from build123d import *

# Parameters (mm, degrees)
SKETCH1_W           = 44
SKETCH1_H           = 16
BOSS_EXTRUDE1_DEPTH = 10
SKETCH2_R           = 1.7
CUT_EXTRUDE1_DEPTH  = 25
SKETCH3_R           = 1.75
CUT_EXTRUDE2_DEPTH  = 25
CHAMFER1_SIZE       = 5
FILLET1_R           = 2
SKETCH4_R           = 3.5
CUT_EXTRUDE3_DEPTH  = 4


with BuildPart() as part:
    # Sketch1 → Boss-Extrude1 (new body)
    with BuildSketch(Plane.XY):
        Rectangle(SKETCH1_W, SKETCH1_H)
    extrude(amount=BOSS_EXTRUDE1_DEPTH)

    # Sketch2 → Cut-Extrude1 (cut)
    with BuildSketch(Plane.XZ.offset(8)):
        with Locations(Location((-10, 5, 0), (0, 0, 270))):
            Circle(SKETCH2_R)
        with Locations(Location((10, 5, 0), (0, 0, 270))):
            Circle(SKETCH2_R)
    extrude(amount=-CUT_EXTRUDE1_DEPTH, mode=Mode.SUBTRACT)

    # Sketch3 → Cut-Extrude2 (cut)
    with BuildSketch(Plane.XY.offset(10)):
        with Locations((-16, 0)):
            Circle(SKETCH3_R)
        with Locations(Location((16, 0, 0), (0, 0, 180))):
            Circle(SKETCH3_R)
    extrude(amount=-CUT_EXTRUDE2_DEPTH, mode=Mode.SUBTRACT)

    # Chamfer1
    chamfer1_edges = [part.edges().sort_by_distance(p)[0] for p in [
        (22, -8, 5),
        (-22, -8, 5),
    ]]
    chamfer(chamfer1_edges, length=CHAMFER1_SIZE)

    # Fillet1
    fillet1_edges = [part.edges().sort_by_distance(p)[0] for p in [
        (22, -3, 5),
        (-17, -8, 5),
        (17, -8, 5),
        (-22, -3, 5),
    ]]
    fillet(fillet1_edges, radius=FILLET1_R)

    # Sketch4 → Cut-Extrude3 (cut)
    with BuildSketch(Plane.XZ.offset(8)):
        with Locations(Location((10, 5, 0), (0, 0, 270))):
            Circle(SKETCH4_R)
        with Locations(Location((-10, 5, 0), (0, 0, 270))):
            Circle(SKETCH4_R)
    extrude(amount=-CUT_EXTRUDE3_DEPTH, mode=Mode.SUBTRACT)


solid = part.part
Source: CAD feature listing. Evaluate the final solid. Frame: model axes, mm. A direction names the side the tool comes from. Round coordinates to 2 decimals unless told otherwise and drop trailing zeros. Loops run counter-clockwise (first coordinate to the right, second up) from the corner with the lowest first, then second, coordinate; pieces in that order, holes last. Notation, with made-up numbers: (8.5, 63.5) -> (56.5, 63.5) arc R24 ccw to (56.5, 88.5) -> close; hole circle Ø11 at (58.25, 16.5). An arc over 180 degrees is marked (long way). Answer as a JSON object with one key per item and string values. Group by question number.
Q1. Section query D-D (z = 5.5). Output: boundary loops of the cut face in (x, y), plus the area to 3 significant figures.
Q2. Section query B-B (x = 10). Output: boundary loops of the cut face in (y, z).
Q3. Access query for faces 4 (the flat face through (-22, 3, 5)), 5 (the flat face through (-9, -4, 3)). Directions: +Z, -Z, +X, -X, +Y, -Y. A direction counts if a zero-diameter tool reaches every point of the face in a straight line with its end or side. Return the directions, or none.
Q4. Contact query for flat-ended pins moving along their axis: P1, Ø2, axis at y = -6, z = 8.5, coming from the -X side; P2, Ø4, axis at x = -10, z = 5, coming from the -Y side. Output: stop coordinate, or through.
Q5. Section query C-C (z = 1). Output: boundary loops of the cut face in (x, y).
Q6. Mould query, pull axis X, two halves, no side actions, for faces 1 (the cylindrical face through (-14.331, 0.526, 5.07)), 2 (the flat face through (0, 0, 0)), 3 (the cylindrical face through (16.93, -7.85, 5.07)). Classes: pulls with the +X half, pulls with the -X half, needs draft (parallel to the pull), parting line crosses it, or undercut.
Q7. Section query A-A (y = 0). Output: boundary loops of the cut face in (x, z), plus the area to 3 significant figures.
Q8. Ray query, line 1 (X direction, y = -3.5, z = 5.25); line 2 (X direction, y = -7.5, z = 5); line 3 (X direction, y = 1, z = 6). Return the intervals inside material, ascending. Write a range as from..to.
Completed:
{
 "1": {"outline": "(-22, -2.17) arc R2 ccw to (-21.41, -3.59) -> (-17.59, -7.41) arc R2 ccw to (-16.17, -8) -> (-13.46, -8) -> (-13.46, -4) -> (-11.62, -4) -> (-11.62, 8) -> (-22, 8) -> close; (-8.38, -4) -> (-6.54, -4) -> (-6.54, -8) -> (6.54, -8) -> (6.54, -4) -> (8.38, -4) -> (8.38, 8) -> (-8.38, 8) -> close; (11.62, -4) -> (13.46, -4) -> (13.46, -8) -> (16.17, -8) arc R2 ccw to (17.59, -7.41) -> (21.41, -3.59) arc R2 ccw to (22, -2.17) -> (22, 8) -> (11.62, 8) -> close; hole circle Ø3.5 at (-16, 0); hole circle Ø3.5 at (16, 0)", "area": "526 mm²"},
 "2": {"outline": "(-8, 0) -> (8, 0) -> (8, 3.3) -> (-4, 3.3) -> (-4, 1.5) -> (-8, 1.5) -> close; (-8, 8.5) -> (-4, 8.5) -> (-4, 6.7) -> (8, 6.7) -> (8, 10) -> (-8, 10) -> close"},
 "3": {"face 4": "+Z, -Z, -X, +Y, -Y", "face 5": "-Y"},
 "4": {"P1": "x = -20", "P2": "y = -4"},
 "5": {"outline": "(-22, -2.17) arc R2 ccw to (-21.41, -3.59) -> (-17.59, -7.41) arc R2 ccw to (-16.17, -8) -> (16.17, -8) arc R2 ccw to (17.59, -7.41) -> (21.41, -3.59) arc R2 ccw to (22, -2.17) -> (22, 8) -> (-22, 8) -> close; hole circle Ø3.5 at (-16, 0); hole circle Ø3.5 at (16, 0)"},
 "6": {"face 1": "undercut", "face 2": "needs draft", "face 3": "pulls with the +X half"},
 "7": {"outline": "(-22, 0) -> (-17.75, 0) -> (-17.75, 10) -> (-22, 10) -> close; (-14.25, 0) -> (14.25, 0) -> (14.25, 10) -> (-14.25, 10) -> close; (17.75, 0) -> (22, 0) -> (22, 10) -> (17.75, 10) -> close; hole circle Ø3.4 at (-10, 5); hole circle Ø3.4 at (10, 5)", "area": "352 mm²"},
 "8": {"line 1": "-21.5..-11.68, -8.32..8.32, 11.68..21.5", "line 2": "-17.49..-13.5, -6.5..6.5, 13.5..17.49", "line 3": "-22..-17.44, -14.56..-11.37, -8.63..8.63, 11.37..14.56, 17.44..22"}
}
